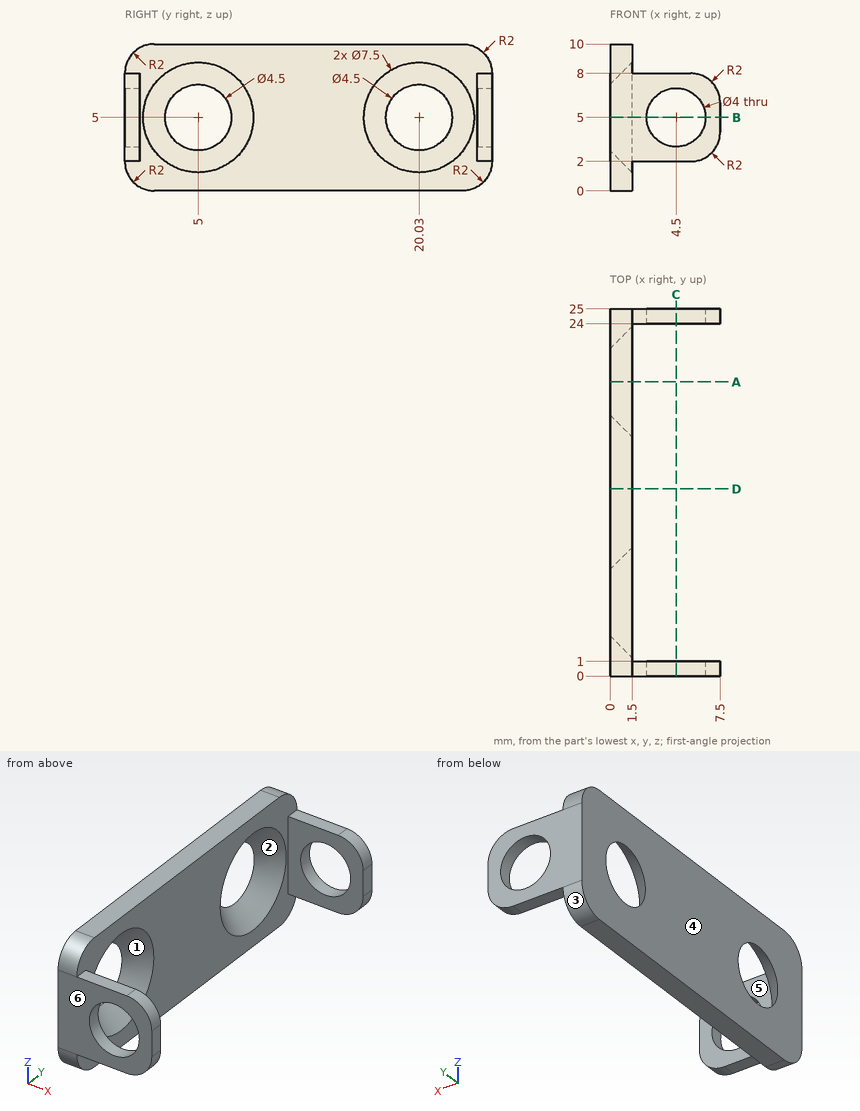
Study the drawing (mm; zero at the part's minimum x, y, z) and answer. A direction names the side the tool comes from. Coordinates: 2 decimals unless noted, no trailing zeros. Order: outer loops, then holes, each group sorted by start corner. A loop starts at its lowest first (then second) coordinate and runs counter-clockwise, first axis right, second up. Notation, with made-up numbers: M -1,42 L 20,42 A29 ccw 20,66 Z; hole C 58.25,-29.5 d9. An arc over 180 degrees is marked long. Use CSV: the item, a comma, the result in double quotes.
Q1. Determine the mould class of the marked faces 1, 2, 3 and 4 for opening direction Z: pulls with the +Z half, pulls with the -Z half, needs draft (parallel to the pull), parting line crosses it, or undercut.
Here are the results:
face 1,"undercut"
face 2,"undercut"
face 3,"pulls with the -Z half"
face 4,"needs draft"
Q2. Section A-A (y = 20.03) is taken. Determine the outline of the cut face in (x, z).
Here are the results:
outline,"M 0,0 L 1.5,0 L 1.5,1.25 L 0,2.75 Z; M 0,7.25 L 1.5,8.75 L 1.5,10 L 0,10 Z"
Q3. Section D-D (y = 12.75) is taken. Determine the outline of the cut face in (x, z), then the cut area to 3 significant figures.
Here are the results:
outline,"M 0,0 L 1.5,0 L 1.5,10 L 0,10 Z"
area,"15.0 mm2"
Q4. A tool of negligible diameter and unlimited length cuts with its end or side. For the marked faces 5 and 6, from which of +Z, -Z, +X, -X, +Y, -Y can it reach the whole face along a straight path? Write none if from no direction.
Here are the results:
face 5,"+Z, -Z, +X"
face 6,"+Z, -Z, +X, -X, -Y"
Q5. Straight lines are drawn through the part: L1, parallel to Z at x = 4.5, y = 0.7; L2, parallel to Y at x = 7, z = 3.75; L3, parallel to X at y = 24.25, z = 5. For each, find the intervals that lie inside material, in ascending order.
Here are the results:
L1,"2 to 3, 7 to 8"
L2,"0 to 1, 24 to 25"
L3,"0 to 2.5, 6.5 to 7.5"
Q6. Section B-B (z = 5) is taken. Determine the outline of the cut face in (x, y), then the cut area to 3 significant figures.
Here are the results:
outline,"M 0,0 L 2.5,0 L 2.5,1 L 1.5,1 L 1.5,1.25 L 0,2.75 Z; M 0,7.25 L 1.5,8.75 L 1.5,16.28 L 0,17.78 Z; M 0,22.28 L 1.5,23.78 L 1.5,24 L 2.5,24 L 2.5,25 L 0,25 Z; M 6.5,0 L 7.5,0 L 7.5,1 L 6.5,1 Z; M 6.5,24 L 7.5,24 L 7.5,25 L 6.5,25 Z"
area,"23.5 mm2"
Q7. Given pin 1 Ø2 at (y, z) = (11, 5) entering from +X; pin 2 Ø0.5 at (x, y) = (4.5, 24.5) entering from -Z; pin 3 Ø1.1 at (x, y) = (4, 24.5) entering from +Z, each flat-ended and moving along its own axis, determine where each tip first touches the part or whether it passes through.
Here are the results:
pin 1,"x = 1.5"
pin 2,"z = 2"
pin 3,"z = 8"
Q8. Section C-C (x = 4.5) is taken. Determine the outline of the cut face in (y, z), then the cut area to 3 significant figures.
Here are the results:
outline,"M 0,2 L 1,2 L 1,3 L 0,3 Z; M 0,7 L 1,7 L 1,8 L 0,8 Z; M 24,2 L 25,2 L 25,3 L 24,3 Z; M 24,7 L 25,7 L 25,8 L 24,8 Z"
area,"4.00 mm2"
